The model under review builds one solid part; all positions refer to its coordinate system, in mm. A direction names the side the tool comes from. Coordinates: 2 decimals unless noted, no trailing zeros. Write each loop counter-clockwise with the first axis right and the second up, starting at its lowest first coordinate (ties: lowest second). Pieces come first, ordered by that corner, then holes. Notation, with made-up numbers: (33, 57.5) - (61, 57.5) arc R19 ccw to (61, 70.5) - close; hole circle Ø5 at (45.25, -6.5). An arc over 180 degrees is marked (long way). Return JSON: item names as keys, results as strings. Group by question number.
(1) For pin 1 Ø3 at (x, y) = (6, -7.5) entering from +Z; pin 2 Ø6 at (x, y) = (6.5, -0.5) entering from -Z, all flat-tipped, find the tip position at first contact; note any pin that passes through.
(2) We need section C-C on z = 1.25. State the section outline as (x, y) points, then the cut area to 3 significant figures.
(3) Tool access review of faces 1 (the face through (12.5, 0, 2)), 2 (the face through (-0.195, 1.013, -0.345)): name each direction out of +Z, -Z, +X, -X, +Y, -Y from which nothing blocks a thin tool from reaching the whole face with its end or side.
(4) To check wall thickness, follow L1, parallel to Z at x = 7.75, y = 0.5; L2, parallel to X at y = 8.75, z = 3.25; L3, parallel to Y at x = 10.25, z = 2. State the ranges of each line that lie inside material, in increasing order. Write a range as from..to.
(5) We need section B-B on x = 0. State the section outline as (y, z) points.
(6) We need section D-D on x = -2.5. State the section outline as (y, z) points, then the cut area to 3 significant figures.
(7) We need section A-A on y = 2.5. State the section outline as (x, z) points, then the cut area to 3 significant figures.
```python
from build123d import *

# Parameters (mm, degrees)
EXTRUDE_1_DEPTH = 4
SKETCH_2_R      = 0.4
EXTRUDE_2_DEPTH = 3.3
SKETCH_3_R      = 1.5
EXTRUDE_3_DEPTH = 0.7


with BuildPart() as part:
    # Эскиз1 → Бобышка-Вытянуть1 (new body)
    with BuildSketch(Plane.XY):
        with BuildLine():
            Line((-8.5, 12.5), (8.5, 12.5))
            ThreePointArc((8.5, 12.5), (11.328427125, 11.328427125), (12.5, 8.5))
            Line((12.5, 8.5), (12.5, -8.5))
            ThreePointArc((12.5, -8.5), (11.328427125, -11.328427125), (8.5, -12.5))
            Line((8.5, -12.5), (-8.5, -12.5))
            ThreePointArc((-8.5, -12.5), (-11.328427125, -11.328427125), (-12.5, -8.5))
            Line((-12.5, -8.5), (-12.5, 8.5))
            ThreePointArc((-12.5, 8.5), (-11.328427125, 11.328427125), (-8.5, 12.5))
        make_face()
    extrude(amount=EXTRUDE_1_DEPTH)

    # Эскиз2 → Бобышка-Вытянуть2 (add)
    with BuildSketch(Plane.XY.offset(4)):
        with Locations((0, 2.5)):
            Circle(SKETCH_2_R)
    extrude(amount=EXTRUDE_2_DEPTH)

    # Эскиз3 → Бобышка-Вытянуть3 (add)
    with BuildSketch(Plane(origin=(0, 0, 0), x_dir=(-1, 0, 0), z_dir=(0, 0, -1))):
        with Locations(Location((0, 2.5, 0), (0, 0, 180))):
            Circle(SKETCH_3_R)
    extrude(amount=EXTRUDE_3_DEPTH)


solid = part.part
```
Ans:
{
 "1": {"pin 1": "z = 4", "pin 2": "z = 0"},
 "2": {"outline": "(-12.5, -8.5) arc R4 ccw to (-8.5, -12.5) - (8.5, -12.5) arc R4 ccw to (12.5, -8.5) - (12.5, 8.5) arc R4 ccw to (8.5, 12.5) - (-8.5, 12.5) arc R4 ccw to (-12.5, 8.5) - close", "area": "611 mm²"},
 "3": {"face 1": "+Z, -Z, +X, +Y, -Y", "face 2": "-Z"},
 "4": {"L1": "0..4", "L2": "-12.49..12.49", "L3": "-12.1..12.1"},
 "5": {"outline": "(-12.5, 0) - (1, 0) - (1, -0.7) - (4, -0.7) - (4, 0) - (12.5, 0) - (12.5, 4) - (2.9, 4) - (2.9, 7.3) - (2.1, 7.3) - (2.1, 4) - (-12.5, 4) - close"},
 "6": {"outline": "(-12.5, 0) - (12.5, 0) - (12.5, 4) - (-12.5, 4) - close", "area": "100 mm²"},
 "7": {"outline": "(-12.5, 0) - (-1.5, 0) - (-1.5, -0.7) - (1.5, -0.7) - (1.5, 0) - (12.5, 0) - (12.5, 4) - (0.4, 4) - (0.4, 7.3) - (-0.4, 7.3) - (-0.4, 4) - (-12.5, 4) - close", "area": "105 mm²"}
}
